from build123d import *

# Parameters (mm, degrees)
F0_W     = 152.4
F0_H     = 101.6
F1_DEPTH = 6.35
F2_R     = 4.78155
F3_DEPTH = 6.35
F5_DEPTH = 6.351
F6_R     = 3.3
F7_DEPTH = 6.351
F9_D     = 11.50874


with BuildPart() as f1:
    # F0 (on Top) → F1 (new body)
    with BuildSketch(Plane.XY):
        Rectangle(F0_W, F0_H)
    extrude(amount=F1_DEPTH)

    # F2 (on face) → F3 (cut, through all)
    with BuildSketch(Plane.XY.offset(6.35)):
        with Locations((-52.3875, 38.1)):
            Circle(F2_R)
        with Locations((52.3875, 38.1)):
            Circle(F2_R)
        with Locations((-52.3875, -38.1)):
            Circle(F2_R)
        with Locations((52.3875, -38.1)):
            Circle(F2_R)
    extrude(amount=-F3_DEPTH, mode=Mode.SUBTRACT)

    # F4 (on face) → F5 (cut, through all)
    with BuildSketch(Plane.XY.offset(6.35)):
        with BuildLine():
            Line((-34.2171942442, -3.5708408817), (-34.13125, -3.571875))
            ThreePointArc((-34.13125, -3.571875), (-34.0882747673, 3.5716164611), (-34.2171942442, -3.5708408817))
        make_face()
        with BuildLine():
            Line((34.13125, -3.571875), (34.2751243473, -3.56897621))
            ThreePointArc((34.2751243473, -3.56897621), (34.0592982266, 3.571150229), (34.13125, -3.571875))
        make_face()
    extrude(amount=-F5_DEPTH, mode=Mode.SUBTRACT)

    # F6 (on face) → F7 (cut, through all)
    with BuildSketch(Plane.XY.offset(6.35)):
        with Locations((-15, 0)):
            Circle(F6_R)
        with Locations((15, 0)):
            Circle(F6_R)
    extrude(amount=-F7_DEPTH, mode=Mode.SUBTRACT)

    # F9 (through all)
    with Locations(Plane(origin=(0, 0, 0), x_dir=(1, 0, 0), z_dir=(0, 0, -1))):
        with Locations((0, 0)):
            Hole(F9_D / 2)


solid = f1.part
The model under review builds one solid part; all positions refer to its coordinate system, in mm. Round coordinates to 2 decimals unless told otherwise and drop trailing zeros. Write each loop counter-clockwise with the first axis right and the second up, starting at its lowest first coordinate (ties: lowest second). Pieces come first, ordered by that corner, then holes. Notation, with made-up numbers: (-38.5, 45.25) - (-0.5, 45.25) arc R31 ccw to (-0.5, 83.25) - close; hole circle Ø1 at (6.25, 33.25). An arc over 180 degrees is marked (long way). One line per item, written item: value. Start each with the question number.
1. The part is to be moulded in two halves that separate along X. For faces 1 (the face through (-1, -11, 0)), 2 (the face through (-76.2, -1, 3)), 3 (the face through (-33.932, 3.566, 3.219)), say which applies: released by +X, released by -X, zero draft, split by the parting line, or undercut.
2. Consider section A-A on y = 38.1. Write out the cut boundary in (x, z), and give its area (3 significant figures).
3. Consider section C-C on x = 15. Write out the cut boundary in (y, z).
4. Consider section B-B on z = 2.5. State how many separate pieces and enclosed holes the cut face has, and give its area (3 significant figures).
5. Consider section D-D on y = 0. Write out the cut boundary in (x, z).
6. To check wall thickness, follow L1, parallel to X at y = 37.5, z = 0.75; L2, parallel to X at y = 37, z = 6; L3, parallel to Y at x = -34.5, z = 3.75. State the ranges of each line that lie inside material, in increasing order. Write a range as from..to.
Checks:
1. face 1: zero draft
1. face 2: released by -X
1. face 3: undercut
2. outline: (-76.2, 0) - (-57.17, 0) - (-57.17, 6.35) - (-76.2, 6.35) - close; (-47.61, 0) - (47.61, 0) - (47.61, 6.35) - (-47.61, 6.35) - close; (57.17, 0) - (76.2, 0) - (76.2, 6.35) - (57.17, 6.35) - close
2. area: 846 mm^2
3. outline: (-50.8, 0) - (-3.3, 0) - (-3.3, 6.35) - (-50.8, 6.35) - close; (3.3, 0) - (50.8, 0) - (50.8, 6.35) - (3.3, 6.35) - close
4. separate pieces: 1
4. enclosed holes: 9
4. area: 14,900 mm^2
5. outline: (-76.2, 0) - (-37.7, 0) - (-37.7, 6.35) - (-76.2, 6.35) - close; (-30.56, 0) - (-18.3, 0) - (-18.3, 6.35) - (-30.56, 6.35) - close; (-11.7, 0) - (-5.75, 0) - (-5.75, 6.35) - (-11.7, 6.35) - close; (5.75, 0) - (11.7, 0) - (11.7, 6.35) - (5.75, 6.35) - close; (18.3, 0) - (30.56, 0) - (30.56, 6.35) - (18.3, 6.35) - close; (37.7, 0) - (76.2, 0) - (76.2, 6.35) - (37.7, 6.35) - close
6. L1: x = -76.2..-57.13, -47.64..47.64, 57.13..76.2
6. L2: x = -76.2..-57.04, -47.73..47.73, 57.04..76.2
6. L3: y = -50.8..-3.55, 3.55..50.8
